The model under review builds one solid part; all positions refer to its coordinate system, in mm. Face numbers are marked on the shaded views. A direction names the side the tool comes from. Give positions to 0.01 mm unless a question says otherwise; leave off trailing zeros. Write each loop counter-clockwise with the first axis right and the second up, starting at its lowest first coordinate (ties: lowest second). Pieces come first, ordered by that corner, then holes. Notation, with made-up numbers: (13.25, 84.5) -> (17.25, 84.5) arc R34 cw to (17.25, 117.5) -> close; hole circle Ø6 at (-11, -40). An arc over 180 degrees is marked (long way). Use CSV: the item, a comma, the result in double quotes.
```python
from build123d import *

# Parameters (mm, degrees)
F1_DEPTH  = 25
F3_DEPTH  = 70
F5_DEPTH  = 10
F6_R      = 7.44
F7_DEPTH  = 35.001
F8_R      = 15
F9_DEPTH  = 10
F11_DEPTH = 20
F13_R     = 35.5
F14_DEPTH = 130
F15_R     = 21.5
F16_DEPTH = 210.001
F18_R     = 35.5
F19_DEPTH = 130
F20_R     = 20.5
F21_DEPTH = 223.001
F22_SIZE  = 2


with BuildPart() as f1:
    # F0 (on Top) → F1 (new body)
    with BuildSketch(Plane.XY):
        with BuildLine():
            Line((90, 106.5), (-90, 106.5))
            ThreePointArc((-90, 106.5), (-97.0710678119, 103.5710678119), (-100, 96.5))
            Line((-100, 96.5), (-100, -96.5))
            ThreePointArc((-100, -96.5), (-97.0710678119, -103.5710678119), (-90, -106.5))
            Line((-90, -106.5), (90, -106.5))
            ThreePointArc((90, -106.5), (97.0710678119, -103.5710678119), (100, -96.5))
            Line((100, -96.5), (100, 96.5))
            ThreePointArc((100, 96.5), (97.0710678119, 103.5710678119), (90, 106.5))
        make_face()
    extrude(amount=-F1_DEPTH)

    # F2 (on face) → F3 (join)
    with BuildSketch(Plane.XY):
        with BuildLine():
            Line((-70, -26.5), (-70, -106.5))
            Line((-70, -106.5), (-55, -106.5))
            Line((-55, -106.5), (-55, -40.4230484541))
            ThreePointArc((-55, -40.4230484541), (4.2462120246, -10.7462120246), (33.9230484541, 48.5))
            Line((33.9230484541, 48.5), (100, 48.5))
            Line((100, 48.5), (100, 63.5))
            Line((100, 63.5), (20, 63.5))
            ThreePointArc((20, 63.5), (-6.3603896932, -0.1396103068), (-70, -26.5))
        make_face()
    extrude(amount=F3_DEPTH)

    # F4 (on face) → F5 (join)
    with BuildSketch(Plane.XY):
        with BuildLine():
            Line((100, -96.5), (100, -46.5))
            Line((100, -46.5), (55, -46.5))
            ThreePointArc((55, -46.5), (44.3933982822, -50.8933982822), (40, -61.5))
            Line((40, -61.5), (40, -106.5))
            Line((40, -106.5), (90, -106.5))
            ThreePointArc((90, -106.5), (97.0710678119, -103.5710678119), (100, -96.5))
        make_face()
    extrude(amount=F5_DEPTH)

    # F6 (on face) → F7 (cut, through all)
    with BuildSketch(Plane.XY.offset(10)):
        with Locations((70, -76.5)):
            Circle(F6_R)
    extrude(amount=-F7_DEPTH, mode=Mode.SUBTRACT)

    # F8 (on face) → F9 (cut)
    with BuildSketch(Plane.XY.offset(10)):
        with Locations((70, -76.5)):
            Circle(F8_R)
    extrude(amount=-F9_DEPTH, mode=Mode.SUBTRACT)

    # F10 (on face) → F11 (cut)
    with BuildSketch(Plane.XY):
        with BuildLine():
            ThreePointArc((91, 29.5), (88.0710678119, 36.5710678119), (81, 39.5))
            Line((81, 39.5), (49.2476414861, 39.5))
            ThreePointArc((49.2476414861, 39.5), (43.2234965193, 37.481834214), (39.630896205, 32.2419354839))
            ThreePointArc((39.630896205, 32.2419354839), (10.6101730553, -17.1101730553), (-38.7419354839, -46.130896205))
            ThreePointArc((-38.7419354839, -46.130896205), (-43.981834214, -49.7234965193), (-46, -55.7476414861))
            Line((-46, -55.7476414861), (-46, -87.5))
            ThreePointArc((-46, -87.5), (-43.0710678119, -94.5710678119), (-36, -97.5))
            Line((-36, -97.5), (21, -97.5))
            ThreePointArc((21, -97.5), (28.0710678119, -94.5710678119), (31, -87.5))
            Line((31, -87.5), (31, -52.5))
            ThreePointArc((31, -52.5), (35.3933982822, -41.8933982822), (46, -37.5))
            Line((46, -37.5), (81, -37.5))
            ThreePointArc((81, -37.5), (88.0710678119, -34.5710678119), (91, -27.5))
            Line((91, -27.5), (91, 29.5))
        make_face()
    extrude(amount=-F11_DEPTH, mode=Mode.SUBTRACT)

    # F13 (on offset) → F14 (join)
    with BuildSketch(Plane.YZ.offset(110)):
        with Locations((56, 70)):
            Circle(F13_R)
    extrude(amount=-F14_DEPTH)

    # F15 (on face) → F16 (cut, through all)
    with BuildSketch(Plane.YZ.offset(110)):
        with Locations((56, 70)):
            Circle(F15_R)
    extrude(amount=-F16_DEPTH, mode=Mode.SUBTRACT)

    # F18 (on offset) → F19 (join)
    with BuildSketch(Plane.XZ.offset(116.5)):
        with Locations((-62.5, 70)):
            Circle(F18_R)
    extrude(amount=-F19_DEPTH)

    # F20 (on face) → F21 (cut, through all)
    with BuildSketch(Plane.XZ.offset(116.5)):
        with Locations((-62.5, 70)):
            Circle(F20_R)
    extrude(amount=-F21_DEPTH, mode=Mode.SUBTRACT)

    # F22
    f22_edges = [f1.edges().sort_by_distance(p)[0] for p in [
        (-83, -116.5, 70),
        (-83, 13.5, 70),
        (-20, 34.5, 70),
        (110, 34.5, 70),
    ]]
    chamfer(f22_edges, length=F22_SIZE)


solid = f1.part
```
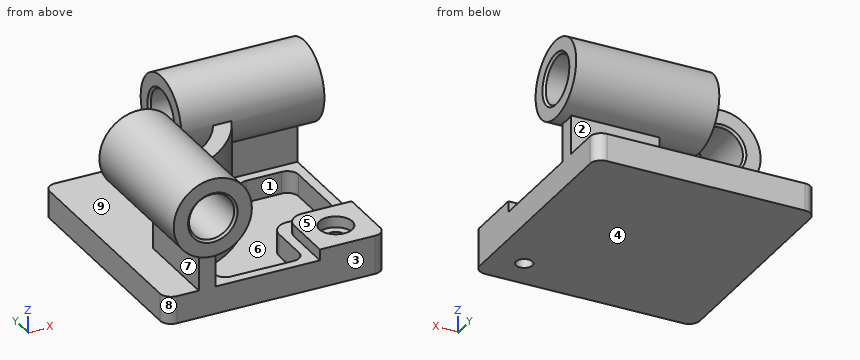
Q1. Insertion check: pin 1 (24 mm diameter, centred on x = 70, y = -76.5, fed in from +Z); pin 2 (5 mm diameter, centred on x = 64.5, z = 58.5, fed in from +Y); pin 3 (10.5 mm diameter, centred on y = -81, z = 10.5, fed in from +X). Each pin has a flat end and moves straight along its axis. Give the tip position at first contact, or say it passes through.
Derived:
pin 1,"stops at z = 0"
pin 2,"stops at y = 90.34"
pin 3,"stops at x = 100"
Q2. Machinability: for the marked faces 5, 6, 7, 8 and 9, which of the approach directions +Z, -Z, +X, -X, +Y, -Y give a long, thin tool a straight path to every point of the face, cutting with its end or side? Answer none if there is none.
Derived:
face 5,"+Z, +X, -Y"
face 6,"none"
face 7,"-X, +Y, -Y"
face 8,"-Z, -X, -Y"
face 9,"-X, +Y"
Q3. The part is to be moulded in two halves that separate along Y. For the marked faces 1, 2, 3 and 4, say which applies: pulls with the +Y half, pulls with the -Y half, needs draft (parallel to the pull), parting line crosses it, or undercut.
Derived:
face 1,"undercut"
face 2,"pulls with the +Y half"
face 3,"pulls with the -Y half"
face 4,"needs draft"
Q4. To check wall thickness, follow probe 1 along Y at (x, z) = (70, -14); probe 2 along Y at (x, z) = (70, 6); probe 3 along Z at (x, y) = (16, 56). State the ranges of each line that lie inside material, in increasing order.
Derived:
probe 1,"y = -106.5 to -83.94, -69.06 to -37.5, 39.5 to 106.5"
probe 2,"y = -106.5 to -91.5, -61.5 to -46.5, 48.5 to 63.5"
probe 3,"z = -25 to 0, 34.5 to 48.5, 91.5 to 105.5"
Q5. Consider section C-C (z = -3). Write out the cut boundary in (x, y), then the cut area to 3 significant figures.
Derived:
outline,"(-100, -96.5) arc R10 ccw to (-90, -106.5) -> (90, -106.5) arc R10 ccw to (100, -96.5) -> (100, 96.5) arc R10 ccw to (90, 106.5) -> (-90, 106.5) arc R10 ccw to (-100, 96.5) -> close; hole (-46, -87.5) arc R10 ccw to (-36, -97.5) -> (21, -97.5) arc R10 ccw to (31, -87.5) -> (31, -52.5) arc R15 cw to (46, -37.5) -> (81, -37.5) arc R10 ccw to (91, -27.5) -> (91, 29.5) arc R10 ccw to (81, 39.5) -> (49.25, 39.5) arc R10 ccw to (39.63, 32.24) arc R114 cw to (-38.74, -46.13) arc R10 ccw to (-46, -55.75) -> close; hole circle Ø14.88 at (70, -76.5)"
area,"32,600 mm2"
Q6. Consider section A-A (x = 70). Write out the cut boundary in (y, z).
Derived:
outline,"(-106.5, -25) -> (-83.94, -25) -> (-83.94, 0) -> (-91.5, 0) -> (-91.5, 10) -> (-106.5, 10) -> close; (-69.06, -25) -> (106.5, -25) -> (106.5, 0) -> (63.5, 0) -> (63.5, 35.3) arc R35.5 ccw (long way) to (48.5, 35.3) -> (48.5, 0) -> (39.5, 0) -> (39.5, -20) -> (-37.5, -20) -> (-37.5, 0) -> (-46.5, 0) -> (-46.5, 10) -> (-61.5, 10) -> (-61.5, 0) -> (-69.06, 0) -> close; hole circle Ø43 at (56, 70)"
Q7. Consider section D-D (y = -12). Write out the cut boundary in (x, z).
Derived:
outline,"(-100, -25) -> (100, -25) -> (100, 0) -> (91, 0) -> (91, -20) -> (15.42, -20) -> (15.42, 0) -> (2.97, 0) -> (2.97, 70) -> (-21.01, 70) -> (-21.01, 0) -> (-100, 0) -> close; circle Ø71 at (-62.5, 70); hole circle Ø41 at (-62.5, 70)"
Q8. Consider section B-B (y = -76.5). Write out the cut boundary in (x, z).
Derived:
outline,"(-100, -25) -> (62.56, -25) -> (62.56, 0) -> (55, 0) -> (55, 10) -> (40, 10) -> (40, 0) -> (31, 0) -> (31, -20) -> (-46, -20) -> (-46, 0) -> (-55, 0) -> (-55, 35.3) arc R35.5 ccw (long way) to (-70, 35.3) -> (-70, 0) -> (-100, 0) -> close; (77.44, -25) -> (100, -25) -> (100, 10) -> (85, 10) -> (85, 0) -> (77.44, 0) -> close; hole circle Ø41 at (-62.5, 70)"
